Can you work these out from the model? Positions are in its coordinate system, mm. Face numbers are marked on the shaded views. A direction names the side the tool comes from. Coordinates: 2 decimals unless noted, no trailing zeros. Order: outer loops, then holes, each group sorted by start corner. A loop starts at its lowest first (then second) coordinate and runs counter-clockwise, first axis right, second up.
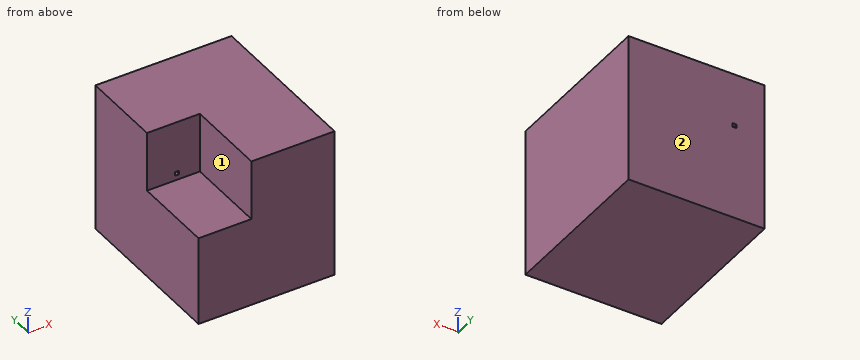
```python
from build123d import *

# Parameters (mm, degrees)
F0_W     = 14.5125519484
F0_H     = 18.9045108855
F0_W_2   = 1.3366825879
F0_H_2   = 1.1457279325
F1_DEPTH = 50.8
F2_DEPTH = 50.8
F3_W     = 16.3383670151
F3_H     = 18.5120366514
F3_W_2   = 1.3366825879
F3_H_2   = 1.1457279325
F4_DEPTH = 25.4


with BuildPart() as f1:
    # F0 (on Front) → F1 (new body)
    with BuildSketch(Plane.XZ):
        Polygon((-42.0100241899, 0), (0, 0), (0, 46.0200719535), (-27.4974722415, 46.0200719535), (-27.4974722415, 27.1155610681), (-42.0100241899, 27.1155610681), align=None)
        with Locations((-34.7537482157, 36.5678165108)):
            Rectangle(F0_W, F0_H)
        with Locations((-32.7487234026, 29.5979715884)):
            Rectangle(F0_W_2, F0_H_2, mode=Mode.SUBTRACT)
    extrude(amount=F1_DEPTH)

    # F0 (on Front) → F2 (join)
    with BuildSketch(Plane.XZ):
        Polygon((-42.0100241899, 0), (0, 0), (0, 46.0200719535), (-27.4974722415, 46.0200719535), (-27.4974722415, 27.1155610681), (-42.0100241899, 27.1155610681), align=None)
        with Locations((-34.7537482157, 36.5678165108)):
            Rectangle(F0_W, F0_H)
        with Locations((-32.7487234026, 29.5979715884)):
            Rectangle(F0_W_2, F0_H_2, mode=Mode.SUBTRACT)
    extrude(amount=F2_DEPTH)

    # F3 (on face) → F4 (cut)
    with BuildSketch(Plane.XZ.offset(50.8)):
        with Locations((-33.8408406824, 36.7640536278)):
            Rectangle(F3_W, F3_H)
        with Locations((-32.7487234026, 29.5979715884)):
            Rectangle(F3_W_2, F3_H_2, mode=Mode.SUBTRACT)
    extrude(amount=-F4_DEPTH, mode=Mode.SUBTRACT)


solid = f1.part
```
1. I'm going to push flat-ended pins straight in: pin 1 (1.3 mm diameter, centred on y = -14, z = 30, fed in from +X); pin 2 (13 mm diameter, centred on x = -35, y = -34, fed in from +Z). Where does each tip first touch, or does it pass through?
Completed:
pin 1: stops at x = 0
pin 2: stops at z = 27.51
2. Please list where these lines run through material, in increasing order: probe 1 along Z at (x, y) = (-33, -12); probe 2 along Y at (x, z) = (-37, 37.5); probe 3 along X at (y, z) = (-44.5, 35).
Completed:
probe 1: z = 0 to 29.03, 30.17 to 46.02
probe 2: y = -25.4 to 0
probe 3: x = -25.67 to 0
3. On a 3-axis mill with a long thin cutter (end or side, diameter ignored), from which of +Z, -Z, +X, -X, +Y, -Y can I reach the whole of each face in a straight line? I mean the marked faces 1 and 2. Say none if no direction works.
Completed:
face 1: +Z, -X, -Y
face 2: +Z, -Z, +X, -X, +Y
4. Imagine slicing it at A-A on x = -29. Please give me the cut outline in (y, z), then the cut area to 3 significant figures.
Completed:
outline: (-50.8, 0) - (0, 0) - (0, 46.02) - (-25.4, 46.02) - (-25.4, 27.51) - (-50.8, 27.51) - close
area: 1,870 mm2
5. Imagine slicing it at B-B on y = -29. Please give me the cut outline in (x, z), then the cut area to 3 significant figures.
Completed:
outline: (-42.01, 0) - (0, 0) - (0, 46.02) - (-25.67, 46.02) - (-25.67, 27.51) - (-42.01, 27.51) - close
area: 1,630 mm2
